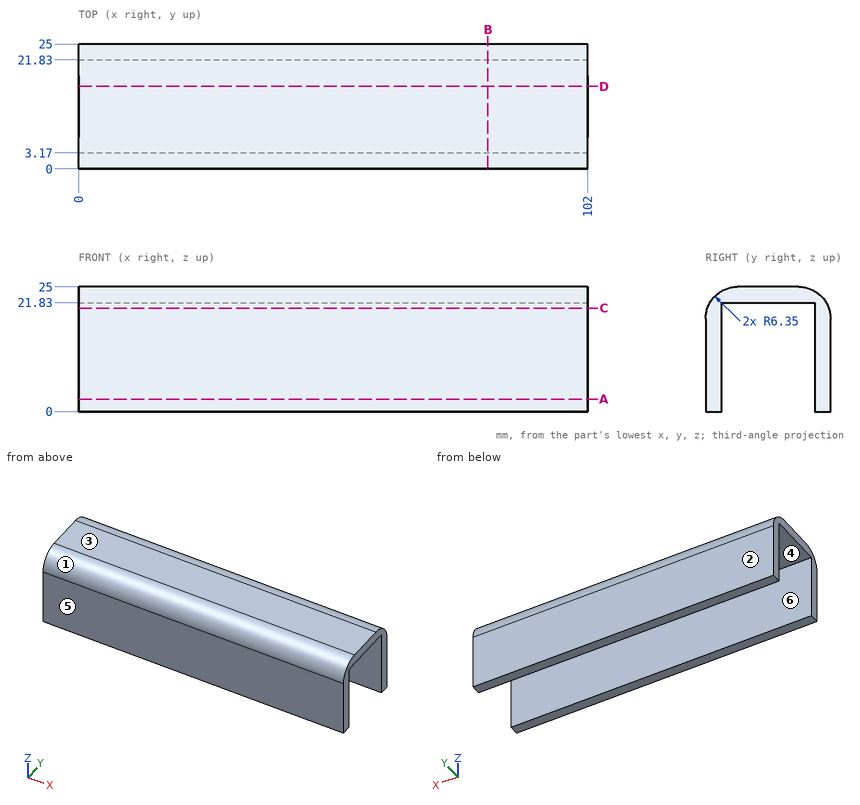
Check sheet for the drawn part. Datum: minimum x, y, z corner. Units: mm. A direction names the side the tool comes from. Round coordinates to 2 decimals unless told otherwise and drop trailing zeros. Order: outer loops, then holes, each group sorted by start corner. A loop starts at its lowest first (then second) coordinate and runs counter-clockwise, first axis right, second up.
(1) Access from +Z, -Z, +X, -X, +Y, -Y to the whole of each face (thin tool, end or side, straight path). Record for the marked faces 5 and 6.
(2) Cross-section at C-C, the plane z = 20.75. Enter the section's corners in (x, y), and give its area (3 significant figures).
(3) Go/stop test with a flat-tipped pin: P1, Ø10, axis at x = 20.5, y = 15.5, coming from the -Z side. Record where the tip stops, or that it passes through.
(4) Cross-section at D-D, the plane y = 16.5. Enter the section's corners in (x, z), and give its area (3 significant figures).
(5) Cross-section at A-A, the plane z = 2.5. Enter the section's corners in (x, y).
(6) Scan lines: probe 1 along Y at (x, z) = (17.5, 2); probe 2 along Z at (x, y) = (28.5, 11); probe 3 along Y at (x, z) = (40.5, 22.25). Record each from-to range of solid material in increasing order.
(7) Draft check along Y on the marked faces 1, 2, 3 and 4. Enter one of: pulls with the +Y half, pulls with the -Y half, needs draft (parallel to the pull), parting line crosses it, or undercut.
(8) Cross-section at B-B, the plane x = 82. Enter the section's corners in (y, z).
Check sheet entries:
1. face 5: +Z, -Z, +X, -X, -Y
1. face 6: -Z, +X, -X
2. outline: (0, 0.36) - (102, 0.36) - (102, 3.17) - (0, 3.17) - close; (0, 21.83) - (102, 21.83) - (102, 24.64) - (0, 24.64) - close
2. area: 574 mm2
3. P1: stops at z = 21.83
4. outline: (0, 21.83) - (102, 21.83) - (102, 25) - (0, 25) - close
4. area: 323 mm2
5. outline: (0, 0) - (102, 0) - (102, 3.17) - (0, 3.17) - close; (0, 21.83) - (102, 21.83) - (102, 25) - (0, 25) - close
6. probe 1: y = 0 to 3.17, 21.83 to 25
6. probe 2: z = 21.83 to 25
6. probe 3: y = 1.12 to 23.88
7. face 1: pulls with the -Y half
7. face 2: pulls with the +Y half
7. face 3: needs draft
7. face 4: undercut
8. outline: (0, 0) - (3.17, 0) - (3.17, 21.83) - (21.83, 21.83) - (21.83, 0) - (25, 0) - (25, 18.65) arc R6.35 ccw to (18.65, 25) - (6.35, 25) arc R6.35 ccw to (0, 18.65) - close
